Read the model definition and answer for the solid it produces. Units are mm, in the model's axes. Coordinates: 2 decimals unless noted, no trailing zeros. Write each loop counter-clockwise with the first axis right and the second up, starting at its lowest first coordinate (ties: lowest second). Pieces come first, ordered by that corner, then holes.
(1) Section C-C on z = 1.45 is taken. State how many separate pieces and enclosed holes the cut face has, then the cut area to 3 significant figures.
(2) Given pin 1 (0.9 mm diameter, centred on x = -30.5, z = 2, fed in from +Y), flat-ended and moving along its own axis, determine where the tip first touches the part or whether it passes through.
(3) Section B-B on y = -17 is taken. Write down the section's boundary in (x, z), then the cut area to 3 significant figures.
(4) Section A-A on x = -12 is taken. Write down the section's boundary in (y, z), then the cut area to 3 significant figures.
(5) Find the intervals of material crossed by probe 1 along X at (y, z) = (-21, 2.8); probe 2 along X at (y, z) = (-29, 1.15); probe 3 along Y at (x, z) = (-45.5, 0.2), in increasing order.
from build123d import *

# Parameters (mm, degrees)
F1_W     = 10.5687566102
F1_H     = 4.3235812336
F1_W_2   = 12.9707455635
F1_H_2   = 6.2451735139
F1_W_3   = 26.4218887314
F1_H_3   = 4.5637749135
F1_W_4   = 17.0541275293
F1_H_4   = 5.7647768408
F2_DEPTH = 3


with BuildPart() as f2:
    # F1 (on face) → F2 (new body)
    with BuildSketch(Plane.XY):
        with BuildLine():
            Line((0, -37.5), (0, 0))
            Line((0, 0), (-37.5, 0))
            ThreePointArc((-37.5, 0), (-10.9834957055, -10.9834957055), (0, -37.5))
        make_face()
        with BuildLine():
            ThreePointArc((-64.0165042945, -10.9834957055), (-51.8506287137, -2.8545175308), (-37.5, 0))
            Line((-37.5, 0), (-75, 0))
            Line((-75, 0), (-64.0165042945, -10.9834957055))
        make_face()
        with BuildLine():
            ThreePointArc((0, -37.5), (-10.9834957055, -10.9834957055), (-37.5, 0))
            ThreePointArc((-37.5, 0), (-51.8506287137, -2.8545175308), (-64.0165042945, -10.9834957055))
            Line((-64.0165042945, -10.9834957055), (-45.3621843147, -29.6378156853))
            Line((-45.3621843147, -29.6378156853), (-57.5412176208, -8.5431112121))
            Line((-57.5412176208, -8.5431112121), (-53.5888726085, -6.2612237553))
            Line((-53.5888726085, -6.2612237553), (-40.3779282428, -29.1432506127))
            Line((-40.3779282428, -29.1432506127), (-43.8513616657, -31.1486383343))
            Line((-43.8513616657, -31.1486383343), (-39.6213203436, -35.3786796564))
            ThreePointArc((-39.6213203436, -35.3786796564), (-36.3519497029, -34.7283614025), (-34.5, -37.5))
            ThreePointArc((-34.5, -37.5), (-34.7283614025, -38.6480502971), (-35.3786796564, -39.6213203436))
            Line((-35.3786796564, -39.6213203436), (-33.8107887229, -41.1892112771))
            Line((-33.8107887229, -41.1892112771), (-32.6696971218, -39.212782648))
            Line((-32.6696971218, -39.212782648), (-28.9253659382, -41.3745732648))
            Line((-28.9253659382, -41.3745732648), (-30.6457075892, -44.3542924108))
            Line((-30.6457075892, -44.3542924108), (-28.5356548637, -46.4643451363))
            Line((-28.5356548637, -46.4643451363), (-27.0296449318, -43.8558594177))
            Line((-27.0296449318, -43.8558594177), (-21.6211660178, -46.9784461747))
            Line((-21.6211660178, -46.9784461747), (-23.9638705494, -51.0361294506))
            Line((-23.9638705494, -51.0361294506), (-21.8538164603, -53.1461835397))
            Line((-21.8538164603, -53.1461835397), (-19.1249452287, -48.4196399192))
            Line((-19.1249452287, -48.4196399192), (-14.1325020374, -51.3020283396))
            Line((-14.1325020374, -51.3020283396), (-17.6337069185, -57.3662930815))
            Line((-17.6337069185, -57.3662930815), (-10.9834957055, -64.0165042945))
            ThreePointArc((-10.9834957055, -64.0165042945), (-2.8545175308, -51.8506287137), (0, -37.5))
        make_face()
        with Locations((-33.1474598497, -30.2986530587)):
            Rectangle(F1_W, F1_H, mode=Mode.SUBTRACT)
        with Locations((-30.7454690337, -22.1318900585)):
            Rectangle(F1_W_2, F1_H_2, mode=Mode.SUBTRACT)
        with Locations((-15.6129342504, -36.9041282684)):
            Rectangle(F1_W_3, F1_H_3, mode=Mode.SUBTRACT)
        with Locations((-28.7037780508, -13.2445273921)):
            Rectangle(F1_W_4, F1_H_4, mode=Mode.SUBTRACT)
        with BuildLine():
            Line((0, -75), (0, -37.5))
            ThreePointArc((0, -37.5), (-2.8545175308, -51.8506287137), (-10.9834957055, -64.0165042945))
            Line((-10.9834957055, -64.0165042945), (0, -75))
        make_face()
        with BuildLine():
            Line((-64.0165042945, -10.9834957055), (-75, 0))
            Line((-75, 0), (-75, -37.5))
            ThreePointArc((-75, -37.5), (-72.1454824692, -23.1493712863), (-64.0165042945, -10.9834957055))
        make_face()
        with BuildLine():
            Line((-45.3621843147, -29.6378156853), (-64.0165042945, -10.9834957055))
            ThreePointArc((-64.0165042945, -10.9834957055), (-72.1454824692, -23.1493712863), (-75, -37.5))
            ThreePointArc((-75, -37.5), (-64.0165042945, -64.0165042945), (-37.5, -75))
            ThreePointArc((-37.5, -75), (-23.1493712863, -72.1454824692), (-10.9834957055, -64.0165042945))
            Line((-10.9834957055, -64.0165042945), (-17.6337069185, -57.3662930815))
            Line((-17.6337069185, -57.3662930815), (-22.659565802, -66.0713360193))
            Line((-22.659565802, -66.0713360193), (-27.6520089933, -63.1889475989))
            Line((-27.6520089933, -63.1889475989), (-21.8538164603, -53.1461835397))
            Line((-21.8538164603, -53.1461835397), (-23.9638705494, -51.0361294506))
            Line((-23.9638705494, -51.0361294506), (-28.1065387995, -58.2114413387))
            Line((-28.1065387995, -58.2114413387), (-33.5150177136, -55.0888545817))
            Line((-33.5150177136, -55.0888545817), (-28.5356548637, -46.4643451363))
            Line((-28.5356548637, -46.4643451363), (-30.6457075892, -44.3542924108))
            Line((-30.6457075892, -44.3542924108), (-34.2097442432, -50.5273849756))
            Line((-34.2097442432, -50.5273849756), (-37.9540754269, -48.3655943588))
            Line((-37.9540754269, -48.3655943588), (-33.8107887229, -41.1892112771))
            Line((-33.8107887229, -41.1892112771), (-35.3786796564, -39.6213203436))
            ThreePointArc((-35.3786796564, -39.6213203436), (-39.6213203436, -39.6213203436), (-39.6213203436, -35.3786796564))
            Line((-39.6213203436, -35.3786796564), (-43.8513616657, -31.1486383343))
            Line((-43.8513616657, -31.1486383343), (-44.3302732551, -31.4251380694))
            Line((-44.3302732551, -31.4251380694), (-45.3621843147, -29.6378156853))
        make_face()
        Polygon((-43.2981931411, -44.1707336622), (-39.3458481288, -46.452621119), (-52.5567924945, -69.3346479764), (-56.5091375068, -67.0527605196), align=None, mode=Mode.SUBTRACT)
        Polygon((-56.1442129559, -47.9534442683), (-61.1366561472, -50.8358326887), (-69.6637199118, -36.066525009), (-64.6712767205, -33.1841365886), align=None, mode=Mode.SUBTRACT)
        Polygon((-48.2395132527, -43.3896637668), (-53.6479921668, -46.5122505238), (-60.1333649485, -35.2792553598), (-54.7248860345, -32.1566686028), align=None, mode=Mode.SUBTRACT)
        Polygon((-41.3984647234, -40.8267736765), (-45.142795907, -42.9885642933), (-50.4271742121, -33.8357525825), (-46.6828430285, -31.6739619657), align=None, mode=Mode.SUBTRACT)
        with BuildLine():
            Line((-37.5, -75), (0, -75))
            Line((0, -75), (-10.9834957055, -64.0165042945))
            ThreePointArc((-10.9834957055, -64.0165042945), (-23.1493712863, -72.1454824692), (-37.5, -75))
        make_face()
        with BuildLine():
            ThreePointArc((-37.5, -75), (-64.0165042945, -64.0165042945), (-75, -37.5))
            Line((-75, -37.5), (-75, -75))
            Line((-75, -75), (-37.5, -75))
        make_face()
    extrude(amount=F2_DEPTH)


solid = f2.part
Response:
1. separate pieces: 1
1. enclosed holes: 13
1. area: 4,560 mm2
2. pin 1: stops at y = 0
3. outline: (-75, 0) - (-52.66, 0) - (-52.66, 3) - (-75, 3) - close; (-47.39, 0) - (0, 0) - (0, 3) - (-47.39, 3) - close
3. area: 209 mm2
4. outline: (-75, 0) - (-39.19, 0) - (-39.19, 3) - (-75, 3) - close; (-34.62, 0) - (0, 0) - (0, 3) - (-34.62, 3) - close
4. area: 211 mm2
5. probe 1: x = -75 to -50.35, -45.08 to -37.23, -24.26 to 0
5. probe 2: x = -75 to -45.73, -40.46 to -38.43, -27.86 to 0
5. probe 3: y = -75 to -57.11, -47.98 to -42.37, -33.72 to -29.4, -20.27 to 0
